For this review, take the finished solid that the model builds, in its own axes (mm). Face numbers are marked on the shaded views. A direction names the side the tool comes from. Give positions to 0.01 mm unless a question says otherwise; leave off trailing zeros. Write each loop counter-clockwise with the first axis right and the second up, starting at its lowest first coordinate (ties: lowest second). Pieces come first, ordered by that corner, then holes.
1) For P1, Ø1.5, axis at x = 17.5, y = 0, coming from the -Z side; P2, Ø10, axis at x = 39.5, z = 6.5, coming from the -Y side; P3, Ø7, axis at x = -20.5, z = -27, coming from the -Y side; P4, Ø2, axis at y = 0.5, z = 38, coming from the -X side, all flat-tipped, find the tip position at first contact; note any pin that passes through.
2) Draft analysis for pull direction Z (two halves, no side actions). For the marked faces 1, 2 and 3, state which applies: pulls with the +Z half, pulls with the -Z half, needs draft (parallel to the pull), parting line crosses it, or undercut.
3) We need section D-D on x = 45. Give the boundary of the cut face in (y, z).
4) Wall thickness on line 1 along X through (y, z) = (-2.5, 0); line 2 along X through (y, z) = (-1.75, 40); line 3 along Z through (x, y) = (-40.5, -1.5): over which ranges is each line inside the solid? List them lowest first.
5) We need section A-A on x = 0. Give the boundary of the cut face in (y, z), and give its area (4 significant figures).
6) We need section B-B on y = -3.5. Give the number of separate pieces and of enclosed holes in the cut face, and give its area (3 significant figures).
7) We need section C-C on z = -14. Give the boundary of the cut face in (x, y).
8) Machinability: for the marked faces 4 and 5, which of the approach directions +Z, -Z, +X, -X, +Y, -Y give a long, thin tool a straight path to every point of the face, cutting with its end or side? Answer none if there is none.
from build123d import *

# Parameters (mm, degrees)
SKETCH2_R           = 62.5
SKETCH2_R_2         = 11.25
SKETCH2_R_3         = 25.25
BOSS_EXTRUDE1_DEPTH = 5
BOSS_EXTRUDE2_START = 3
SKETCH1_R           = 62.5
BOSS_EXTRUDE2_DEPTH = 3


with BuildPart() as part:
    # Sketch2 → Boss-Extrude1 (new body)
    with BuildSketch(Plane(origin=(0, 0, 0), x_dir=(1, 0, 0), z_dir=(0, 1, 0))):
        with Locations(Location((0, 0, 0), (0, 0, 270))):
            Circle(SKETCH2_R)
        with Locations(Location((0, 37.5, 0), (0, 0, 270))):
            Circle(SKETCH2_R_2, mode=Mode.SUBTRACT)
        with Locations(Location((22.041946961, 30.338137289, 0), (0, 0, 270))):
            Circle(SKETCH2_R_2, mode=Mode.SUBTRACT)
        with Locations(Location((35.664619361, 11.588137289, 0), (0, 0, 270))):
            Circle(SKETCH2_R_2, mode=Mode.SUBTRACT)
        with Locations(Location((35.664619361, -11.588137289, 0), (0, 0, 270))):
            Circle(SKETCH2_R_2, mode=Mode.SUBTRACT)
        with Locations(Location((22.041946961, -30.338137289, 0), (0, 0, 270))):
            Circle(SKETCH2_R_2, mode=Mode.SUBTRACT)
        with Locations(Location((0, -37.5, 0), (0, 0, 270))):
            Circle(SKETCH2_R_2, mode=Mode.SUBTRACT)
        with Locations(Location((-22.041946961, -30.338137289, 0), (0, 0, 270))):
            Circle(SKETCH2_R_2, mode=Mode.SUBTRACT)
        with Locations(Location((-35.664619361, -11.588137289, 0), (0, 0, 270))):
            Circle(SKETCH2_R_2, mode=Mode.SUBTRACT)
        with Locations(Location((-35.664619361, 11.588137289, 0), (0, 0, 270))):
            Circle(SKETCH2_R_2, mode=Mode.SUBTRACT)
        with Locations(Location((-22.041946961, 30.338137289, 0), (0, 0, 270))):
            Circle(SKETCH2_R_2, mode=Mode.SUBTRACT)
        with Locations(Location((0, 0, 0), (0, 0, 270))):
            Circle(SKETCH2_R_3, mode=Mode.SUBTRACT)
    extrude(amount=-BOSS_EXTRUDE1_DEPTH)

    # Sketch1 → Boss-Extrude2 (add)
    with BuildSketch(Plane(origin=(0, 0, 0), x_dir=(1, 0, 0), z_dir=(0, 1, 0)).offset(BOSS_EXTRUDE2_START)):
        with Locations(Location((0, 0, 0), (0, 0, 270))):
            Circle(SKETCH1_R)
    extrude(amount=-BOSS_EXTRUDE2_DEPTH)


solid = part.part
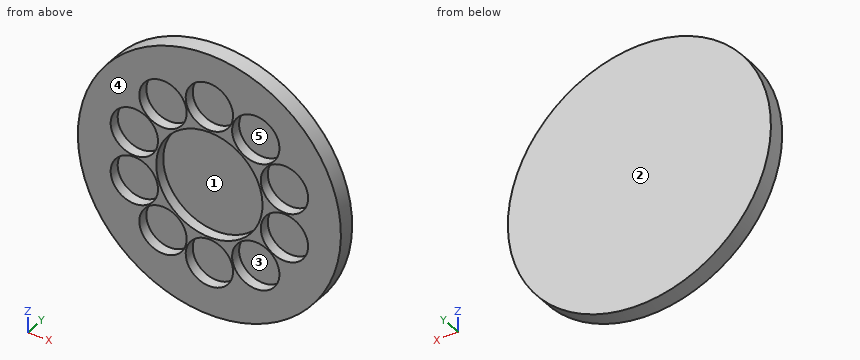
Results list:
1. P1: stops at z = -60.21
1. P2: stops at y = -5
1. P3: stops at y = 0
1. P4: stops at x = -50.37
2. face 1: undercut
2. face 2: needs draft
2. face 3: undercut
3. outline: (-5, -43.37) - (3, -43.37) - (3, 43.37) - (-5, 43.37) - (-5, 17.87) - (0, 17.87) - (0, 5.31) - (-5, 5.31) - (-5, -5.31) - (0, -5.31) - (0, -17.87) - (-5, -17.87) - close
4. line 1: x = -62.5 to -25.25, 25.25 to 62.5
4. line 2: x = -48.02 to -27.8, -16.28 to -10.97, 10.97 to 16.28, 27.8 to 48.02
4. line 3: z = -47.6 to -21.75, -1.43 to 1.43, 21.75 to 47.6
5. outline: (-5, -62.5) - (3, -62.5) - (3, 62.5) - (-5, 62.5) - (-5, 48.75) - (0, 48.75) - (0, 26.25) - (-5, 26.25) - (-5, 25.25) - (0, 25.25) - (0, -25.25) - (-5, -25.25) - (-5, -26.25) - (0, -26.25) - (0, -48.75) - (-5, -48.75) - close
5. area: 522.5 mm2
6. separate pieces: 1
6. enclosed holes: 11
6. area: 6,290 mm2
7. outline: (-60.91, -5) - (-46.65, -5) - (-46.65, 0) - (-24.68, 0) - (-24.68, -5) - (-21.01, -5) - (-21.01, 0) - (21.01, 0) - (21.01, -5) - (24.68, -5) - (24.68, 0) - (46.65, 0) - (46.65, -5) - (60.91, -5) - (60.91, 3) - (-60.91, 3) - close
8. face 4: +Z, -Z, +X, -X, -Y
8. face 5: -Y
